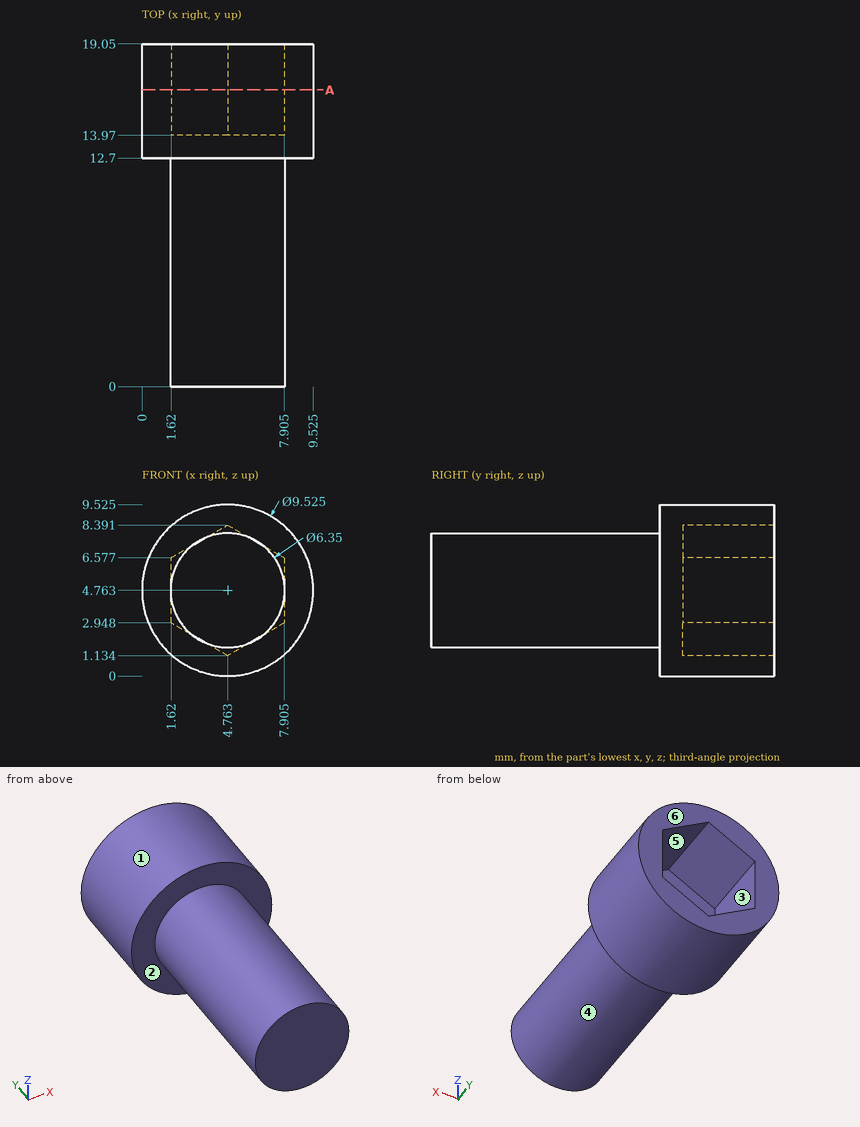
Can you work these out from the drawing? Everything is in mm from the part's minimum corner. A direction names the side the tool comes from. Coordinates: 2 decimals unless noted, no trailing zeros. Loops run counter-clockwise (first coordinate to the right, second up) from the corner with the lowest first, then second, coordinate; pieces in that order, holes last. Notation, with made-up numbers: M -14.75,-25.5 L 9.25,-25.5 A15 ccw 9.25,-8.5 Z; hole C -5.75,5.25 d4. An arc over 180 degrees is marked long. Put each result on its own line as item: value. Start each with the question number.
(1) Suppose I cut it at A-A on y = 16.5. Please give me the cut outline in (x, z) (1 decimal).
(2) For the marked faces 1, 2 and 3, which set-ups out of +Z, -Z, +X, -X, +Y, -Y let a thin tool reach every point of the face, with its end or its side?
(3) I need wall thicknesses on line 1 (Y direction, x = 3.25, z = 1.25); line 2 (Y direction, x = 1.75, z = 3); line 3 (Z direction, x = 7, y = 15.5) (1 decimal). Which ranges of each line are inside material? Lowest first, please. Write a range as from..to.
(4) Thinking about a two-plate mould opening in X: for the marked faces 4, 5 and 6, which applies, pulls with the +X half, pulls with the -X half, needs draft (parallel to the pull), parting line crosses it, or undercut?
(5) Will these pins go through, and if not, where does the flat tip stop? P1, Ø2, axis at x = 2, y = 4, coming from the -Z side; P2, Ø1.5, axis at x = 2, y = 2.5, coming from the +Z side; P3, Ø5, axis at x = 1.5, y = 16.5, coming from the -Z side.
Solutions:
1. outline: C 4.8,4.8 d9.5; hole M 1.6,2.9 L 4.8,1.1 L 7.9,2.9 L 7.9,6.6 L 4.8,8.4 L 1.6,6.6 Z
2. face 1: +Y, -Y
2. face 2: -Y
2. face 3: +Y
3. line 1: y = 12.7..19.05
3. line 2: y = 12.7..13.97
3. line 3: z = 0.6..2.4, 7.1..9
4. face 4: parting line crosses it
4. face 5: undercut
4. face 6: needs draft
5. P1: stops at z = 2.12
5. P2: stops at z = 7.22
5. P3: stops at z = 0.06
